For this review, take the finished solid that the model builds, in its own axes (mm). A direction names the side the tool comes from. Coordinates: 2 decimals unless noted, no trailing zeros. Order: outer loops, then holes, each group sorted by start corner. A loop starts at its lowest first (then second) coordinate and runs counter-clockwise, first axis right, second up. Notation, with made-up numbers: (73.5, -31.5) -> (121.5, -31.5) arc R5 ccw to (121.5, -24.5) -> close; hole circle Ø7 at (81.5, 26.5). An arc over 180 degrees is marked (long way). Write item = value, one per line. Start each with the question number.
1) Consider section D-D on y = 90. Give the boundary of the cut face in (x, z), and give its area (3 significant figures).
2) Draft analysis for pull direction X (two halves, no side actions). For faces 1 (the face through (61.237, 91, 18)), 2 (the face through (29.313, 118.578, 1.479)), 3 (the face through (20.18, 137.28, 1.48)), state which applies: +X half, -X half, draft (parallel to the pull), parting line (faces both ways), or undercut.
3) Consider section B-B on y = 110.5. Give the boundary of the cut face in (x, z).
4) Machinability: for faces 4 (the face through (50.84, 29.09, 1.48)), 5 (the face through (33.796, 132.935, 1.479)), 6 (the face through (41.54, 42.72, 1.48)), which of the approach directions +Z, -Z, +X, -X, +Y, -Y give a long, thin tool a straight path to every point of the face, cutting with its end or side? Answer none if there is none.
5) Consider section A-A on z = 28. Give the boundary of the cut face in (x, y).
6) Insertion check: pin 1 Ø20.5 at (x, y) = (50, 89) entering from +Z; pin 2 Ø10 at (y, z) = (76, 23.5) entering from -X. Each pin has a flat end and moves straight along its axis. Give the tip position at first contact, or say it passes through.
7) Wall thickness on probe 1 along Z at (x, y) = (5, 110); probe 2 along X at (y, z) = (101, 4); probe 3 along Y at (x, z) = (49.5, 1): over which ranges is each line inside the solid? List them lowest first. Write a range as [from, to].
8) Consider section C-C on x = 63.5. Give the boundary of the cut face in (y, z), and give its area (3 significant figures).
from build123d import *

# Parameters (mm, degrees)
BOSS_EXTRUDE2_DEPTH = 3
BOSS_EXTRUDE3_DEPTH = 30.5


with BuildPart() as part:
    # Sketch1 → Boss-Extrude2 (new body)
    with BuildSketch(Plane.XY):
        with BuildLine():
            Line((13.275380686, 31.205054945), (14.898132017, 31.200709019))
            Line((14.898132017, 31.200709019), (15.525048851, 29.699024681))
            Line((15.525048851, 29.699024681), (13.895725818, 29.703388206))
            ThreePointArc((13.895725818, 29.703388206), (18.832488619, 18.980593631), (24.505317159, 8.628349101))
            ThreePointArc((24.505317159, 8.628349101), (24.86546573, 8.055516696), (25.253864185, 7.501449375))
            ThreePointArc((25.253864185, 7.501449375), (31.492395544, 2.238754737), (39.432559358, 0.349567888))
            Line((39.432559358, 0.349567888), (54.166964146, 0.349567888))
            ThreePointArc((54.166964146, 0.349567888), (65.260793251, 5.589158017), (69.367502095, 17.15035568))
            ThreePointArc((69.367502095, 17.15035568), (64.201860596, 26.406348327), (54.004278297, 29.298850229))
            ThreePointArc((54.004278297, 29.298850229), (50.794421974, 29.086613139), (47.592527294, 28.776624992))
            ThreePointArc((47.592527294, 28.776624992), (46.406851761, 28.931308018), (45.428630625, 29.618939254))
            Line((45.428630625, 29.618939254), (43.664188783, 29.623664644))
            Line((43.664188783, 29.623664644), (43.305228514, 31.124631363))
            Line((43.305228514, 31.124631363), (44.814654419, 31.120588936))
            ThreePointArc((44.814654419, 31.120588936), (41.465663123, 42.879415537), (34.373869876, 52.838944354))
            ThreePointArc((34.373869876, 52.838944354), (31.77008993, 61.224226607), (35.075221649, 69.358643168))
            ThreePointArc((35.075221649, 69.358643168), (36.634181143, 70.853545892), (38.565369315, 71.820810645))
            ThreePointArc((38.565369315, 71.820810645), (41.657810048, 72.796166819), (44.793456308, 73.622140114))
            Line((44.793456308, 73.622140114), (49.906358238, 74.39986774))
            Line((49.906358238, 74.39986774), (72.499029275, 78.04718712))
            Line((72.499029275, 78.04718712), (72.499029275, 112.666688298))
            Line((72.499029275, 112.666688298), (64.965959637, 108.371234093))
            ThreePointArc((64.965959637, 108.371234093), (55.215260948, 103.529752912), (44.974426149, 99.836330705))
            ThreePointArc((44.974426149, 99.836330705), (32.918019246, 103.856141001), (28.925028873, 115.921456997))
            Line((28.925028873, 115.921456997), (29.712339951, 121.309986069))
            ThreePointArc((29.712339951, 121.309986069), (31.21062393, 126.530705767), (34.041547196, 131.166074417))
            ThreePointArc((34.041547196, 131.166074417), (34.181825554, 131.336695356), (34.323954998, 131.505777418))
            ThreePointArc((34.323954998, 131.505777418), (35.033278252, 132.297306273), (35.783119531, 133.050562846))
            ThreePointArc((35.783119531, 133.050562846), (35.963964723, 133.201914626), (36.140056994, 133.358770791))
            Line((36.140056994, 133.358770791), (31.386106103, 132.498519796))
            ThreePointArc((31.386106103, 132.498519796), (20.056581392, 137.416407931), (16.627117574, 149.281589422))
            ThreePointArc((16.627117574, 149.281589422), (15.570836478, 149.356522247), (14.534507264, 149.138883925))
            ThreePointArc((14.534507264, 149.138883925), (11.661008479, 146.078583559), (9.194011926, 142.682061573))
            ThreePointArc((9.194011926, 142.682061573), (7.06412615, 138.77022346), (5.473593477, 134.609803211))
            ThreePointArc((5.473593477, 134.609803211), (1.252330233, 82.294620281), (13.275380686, 31.205054945))
        make_face()
    extrude(amount=BOSS_EXTRUDE2_DEPTH)

    # Sketch2 → Boss-Extrude3 (add)
    with BuildSketch(Plane.XY.offset(3)):
        with BuildLine():
            Line((61.236736711, 76.229023262), (61.236736711, 106.35376845))
            ThreePointArc((61.236736711, 106.35376845), (63.112611761, 107.341680879), (64.965959637, 108.371234093))
            Line((64.965959637, 108.371234093), (72.499029275, 112.666688298))
            Line((72.499029275, 112.666688298), (72.499029275, 78.04718712))
            Line((72.499029275, 78.04718712), (61.236736711, 76.229023262))
        make_face()
    extrude(amount=BOSS_EXTRUDE3_DEPTH)


solid = part.part
Answer sheet:
q1.outline = (0.85, 0) -> (72.5, 0) -> (72.5, 33.5) -> (61.24, 33.5) -> (61.24, 3) -> (0.85, 3) -> close
q1.area = 558 mm2
q2.face_1 = -X half
q2.face_2 = +X half
q2.face_3 = undercut
q3.outline = (1.48, 0) -> (29.18, 0) -> (29.18, 3) -> (1.48, 3) -> close; (68.7, 0) -> (72.5, 0) -> (72.5, 33.5) -> (68.7, 33.5) -> close
q4.face_4 = +Z, -Z
q4.face_5 = +Z, -Z, +Y
q4.face_6 = +Z, -Z, +X
q5.outline = (61.24, 76.23) -> (72.5, 78.05) -> (72.5, 112.67) -> (64.97, 108.37) arc R94.94 cw to (61.24, 106.35) -> close
q6.pin_1 = 3
q6.pin_2 = 61.24
q7.probe_1 = [0, 3]
q7.probe_2 = [61.24, 72.5]
q7.probe_3 = [0.35, 28.97], [74.34, 101.31]
q8.outline = (3.92, 0) -> (26.93, 0) -> (26.93, 3) -> (3.92, 3) -> close; (76.59, 0) -> (107.55, 0) -> (107.55, 33.5) -> (76.59, 33.5) -> close
q8.area = 1,110 mm2
